Could you check a few things on this model? Use its own coordinates, in mm. Face numbers are marked on the shaded views. A direction names the side the tool comes from. Round coordinates to 2 decimals unless told otherwise and drop trailing zeros. Loops run counter-clockwise (first coordinate to the right, second up) from the corner with the lowest first, then second, coordinate; pieces in that order, holes last. Notation, with made-up numbers: (-6.75, 57) - (38.25, 57) arc R31 cw to (38.25, 86) - close; hole circle Ø1 at (76, -39). An arc over 180 degrees is marked (long way). Use one line per item in the form item = value.
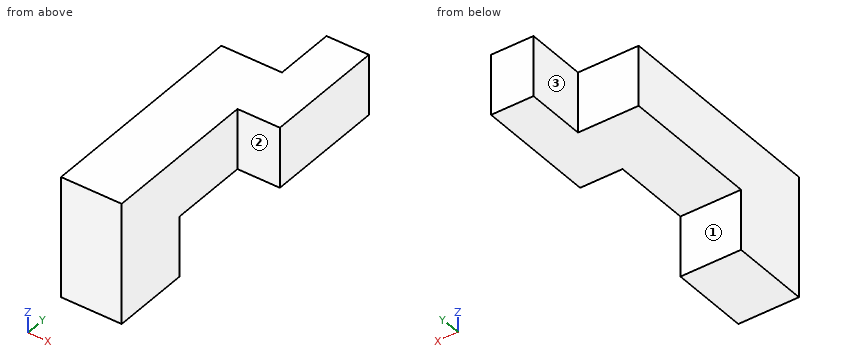
```python
from build123d import *

# Parameters (mm, degrees)
F0_W     = 25.4
F0_H     = 25.4
F1_DEPTH = 17.78
F2_DEPTH = 43.18
F3_W     = 25.4
F3_H     = 25.4
F4_DEPTH = 66.04
F5_W     = 25.4
F5_H     = 33.02
F6_DEPTH = 25.4


with BuildPart() as f1:
    # F0 (on Right) → F1 (new body)
    with BuildSketch(Plane.YZ):
        with Locations((58.3694662571, -26.3017169727)):
            Rectangle(F0_W, F0_H)
    extrude(amount=-F1_DEPTH)

    # F0 (on Right) → F2 (join)
    with BuildSketch(Plane.YZ):
        with Locations((32.9694662571, -26.3017169727)):
            Rectangle(F0_W, F0_H)
    extrude(amount=-F2_DEPTH)

    # F3 (on face) → F4 (join)
    with BuildSketch(Plane.XZ.offset(-20.2694662571)):
        with Locations((-30.48, -26.3017169727)):
            Rectangle(F3_W, F3_H)
    extrude(amount=F4_DEPTH)

    # F5 (on face) → F6 (join)
    with BuildSketch(Plane(origin=(0, 0, -39.0017169727), x_dir=(1, 0, 0), z_dir=(0, 0, -1))):
        with Locations((-30.48, 29.2605337429)):
            Rectangle(F5_W, F5_H)
    extrude(amount=F6_DEPTH)


solid = f1.part
```
1. Please list where these lines run through material, in increasing order: line 1 along Z through (x, y) = (-24, 34); line 2 along X through (y, z) = (-24.5, -41); line 3 along Y through (x, z) = (-25.5, -52).
Solution:
line_1 = -39 to -13.6
line_2 = -43.18 to -17.78
line_3 = -45.77 to -12.75
2. For P1, Ø7.5, axis at x = -36.5, z = -55.5, coming from the +Y side; P2, Ø8, axis at x = -7, z = -28, coming from the -Y side; P3, Ø6, axis at y = -10.5, z = -42.5, coming from the +X side, each with a flat end and sliding along its axis, tell me the tip position at first contact or that it passes through.
Solution:
P1 = -12.75
P2 = 20.27
P3 = -17.78
3. On a 3-axis mill with a long thin cutter (end or side, diameter ignored), from which of +Z, -Z, +X, -X, +Y, -Y can I reach the whole of each face in a straight line? I mean the marked faces 1, 2 and 3. Say none if no direction works.
Solution:
face_1 = -Z, +X, -X, +Y
face_2 = +Z, -Z, +X, -Y
face_3 = +Z, -Z, -X, +Y
4. If we section it at C-C, the plane y = -20: Write out the boundary of the cut face in (x, z), plus the area to 3 significant figures.
Solution:
outline = (-43.18, -64.4) - (-17.78, -64.4) - (-17.78, -13.6) - (-43.18, -13.6) - close
area = 1,290 mm^2
5. If we section it at A-A, the plane z = -17: Write out the boundary of the cut face in (x, y).
Solution:
outline = (-43.18, -45.77) - (-17.78, -45.77) - (-17.78, 20.27) - (0, 20.27) - (0, 71.07) - (-17.78, 71.07) - (-17.78, 45.67) - (-43.18, 45.67) - close
6. If we section it at B-B, the plane x = -29: Write out the boundary of the cut face in (y, z), plus the area to 3 significant figures.
Solution:
outline = (-45.77, -64.4) - (-12.75, -64.4) - (-12.75, -39) - (45.67, -39) - (45.67, -13.6) - (-45.77, -13.6) - close
area = 3,160 mm^2
7. If we section it at D-D, the plane x = -8: Write out the boundary of the cut face in (y, z).
Solution:
outline = (20.27, -39) - (71.07, -39) - (71.07, -13.6) - (20.27, -13.6) - close
